Source: CAD feature listing. Evaluate the final solid. Frame: model axes, mm. Give positions to 0.01 mm unless a question says otherwise; leave off trailing zeros. Order: outer loops, then holes, each group sorted by start corner. A loop starts at its lowest first (then second) coordinate and runs counter-clockwise, first axis right, second up. Notation, with made-up numbers: M -7,66.5 L 2,66.5 A20 cw 2,93.5 Z; hole C 57,71.25 d6. An arc over 180 degrees is marked long. Answer as a JSON object with one key per item and string values. Group by question number.
1. Section query C-C (x = -66.5). Output: boundary loops of the cut face in (y, z), plus the area to 3 significant figures.
2. Material intervals for L1, parallel to Y at x = 31.5, z = 1.75; L2, parallel to Y at x = 16, z = 1.35; L3, parallel to Y at x = 50, z = 0.55, sorted ascending. Write a range as [from, to].
3. Pin query (flat end, axial travel): P1, Ø1.5, axis at y = 150, z = 1.5, coming from the -X side; P2, Ø1.7, axis at y = 218, z = 1, coming from the -X side. Return the tip coordinate at first contact, or that it passes through.
4. Section query A-A (y = 34.03). Output: boundary loops of the cut face in (x, z) (3 decimals).
5. Section query B-B (z = 1.5). Count the separate pieces of the cut face and the enclosed holes in it, plus the area to 3 significant figures.
from build123d import *

# Parameters (mm, degrees)
MODEL_R             = 3.6
MODEL_R_2           = 2.5
BOSS_EXTRUDE1_DEPTH = 3


with BuildPart() as part:
    # Model → Boss-Extrude1 (new body)
    with BuildSketch(Plane.XY):
        with BuildLine():
            Line((-86.64, 0), (86.64, 0))
            ThreePointArc((86.64, 0), (89.015878785, 0.984121215), (90, 3.36))
            Line((90, 3.36), (90, 217.83))
            ThreePointArc((90, 217.83), (87.167722574, 224.667722574), (80.33, 227.5))
            Line((80.33, 227.5), (-19.67, 227.5))
            ThreePointArc((-19.67, 227.5), (-25.584006957, 225.942971908), (-29.964579281, 221.67560728))
            Line((-29.964579281, 221.67560728), (-86.618767522, 127.387204203))
            ThreePointArc((-86.618767522, 127.387204203), (-89.126906327, 120.031940724), (-90, 112.31))
            Line((-90, 112.31), (-90, 3.36))
            ThreePointArc((-90, 3.36), (-89.015878785, 0.984121215), (-86.64, 0))
        make_face()
        with Locations((-75.285, 13.33)):
            Circle(MODEL_R, mode=Mode.SUBTRACT)
        with Locations((-7.295, 209.94)):
            Circle(MODEL_R_2, mode=Mode.SUBTRACT)
        with Locations((-7.295, 189.94)):
            Circle(MODEL_R_2, mode=Mode.SUBTRACT)
        with Locations((-7.295, 169.94)):
            Circle(MODEL_R_2, mode=Mode.SUBTRACT)
        with Locations((-35.285, 113.03)):
            Circle(MODEL_R_2, mode=Mode.SUBTRACT)
        with Locations((-75.285, 113.03)):
            Circle(MODEL_R_2, mode=Mode.SUBTRACT)
        with Locations((75.315, 13.33)):
            Circle(MODEL_R, mode=Mode.SUBTRACT)
        with Locations((0, 13.33)):
            Circle(MODEL_R, mode=Mode.SUBTRACT)
        with Locations((56.355, 34.03)):
            Circle(MODEL_R_2, mode=Mode.SUBTRACT)
        with Locations((53.705, 189.94)):
            Circle(MODEL_R_2, mode=Mode.SUBTRACT)
        with Locations((73.365, 165.98)):
            Circle(MODEL_R_2, mode=Mode.SUBTRACT)
        with Locations((73.365, 145.98)):
            Circle(MODEL_R_2, mode=Mode.SUBTRACT)
        with Locations((52.865, 145.98)):
            Circle(MODEL_R_2, mode=Mode.SUBTRACT)
        with Locations((56.355, 129.03)):
            Circle(MODEL_R_2, mode=Mode.SUBTRACT)
        with Locations((75.315, 113.03)):
            Circle(MODEL_R_2, mode=Mode.SUBTRACT)
        with Locations((35.315, 113.03)):
            Circle(MODEL_R_2, mode=Mode.SUBTRACT)
        with BuildLine():
            Line((-26.095, 100.21), (-26.095, 109.21))
            ThreePointArc((-26.095, 109.21), (-23.555, 111.75), (-21.015, 109.21))
            Line((-21.015, 109.21), (-21.015, 100.21))
            ThreePointArc((-21.015, 100.21), (-23.555, 97.67), (-26.095, 100.21))
        make_face(mode=Mode.SUBTRACT)
        with BuildLine():
            Line((-26.095, 147.35), (-26.095, 156.35))
            ThreePointArc((-26.095, 156.35), (-23.555, 158.89), (-21.015, 156.35))
            Line((-21.015, 156.35), (-21.015, 147.35))
            ThreePointArc((-21.015, 147.35), (-23.555, 144.81), (-26.095, 147.35))
        make_face(mode=Mode.SUBTRACT)
        with BuildLine():
            Line((21.045, 100.21), (21.045, 109.21))
            ThreePointArc((21.045, 109.21), (23.585, 111.75), (26.125, 109.21))
            Line((26.125, 109.21), (26.125, 100.21))
            ThreePointArc((26.125, 100.21), (23.585, 97.67), (21.045, 100.21))
        make_face(mode=Mode.SUBTRACT)
        with BuildLine():
            Line((21.045, 147.35), (21.045, 156.35))
            ThreePointArc((21.045, 156.35), (23.585, 158.89), (26.125, 156.35))
            Line((26.125, 156.35), (26.125, 147.35))
            ThreePointArc((26.125, 147.35), (23.585, 144.81), (21.045, 147.35))
        make_face(mode=Mode.SUBTRACT)
        with BuildLine():
            Line((27.205, 216.97), (27.205, 219.09))
            ThreePointArc((27.205, 219.09), (27.626766235, 220.108233765), (28.645, 220.53))
            Line((28.645, 220.53), (37.765, 220.53))
            ThreePointArc((37.765, 220.53), (38.783233765, 220.108233765), (39.205, 219.09))
            Line((39.205, 219.09), (39.205, 216.97))
            ThreePointArc((39.205, 216.97), (38.783233765, 215.951766235), (37.765, 215.53))
            Line((37.765, 215.53), (28.645, 215.53))
            ThreePointArc((28.645, 215.53), (27.626766235, 215.951766235), (27.205, 216.97))
        make_face(mode=Mode.SUBTRACT)
        with BuildLine():
            Line((76.385, 175.96), (75.817986625, 175.249714613))
            add(Edge.make_bspline(
                [(70.912013375, 175.249714613), (70.912013375, 172.796727988), (73.365, 172.796727988), (75.817986625, 172.796727988), (75.817986625, 175.249714613)],
                knots=[3.141592654, 3.141592654, 3.141592654, 4.71238898, 4.71238898, 6.283185307, 6.283185307, 6.283185307], degree=2, weights=[1, 0.707106781, 1, 0.707106781, 1]))
            Line((70.912013375, 175.249714613), (69.945, 176.461071346))
            Line((69.945, 176.461071346), (67.475, 176.461071346))
            ThreePointArc((67.475, 176.461071346), (66.301202743, 176.947274089), (65.815, 178.121071346))
            Line((65.815, 178.121071346), (65.815, 190.45))
            ThreePointArc((65.815, 190.45), (66.301202743, 191.623797257), (67.475, 192.11))
            Line((67.475, 192.11), (78.855, 192.11))
            ThreePointArc((78.855, 192.11), (80.028797257, 191.623797257), (80.515, 190.45))
            Line((80.515, 190.45), (80.515, 177.62))
            ThreePointArc((80.515, 177.62), (80.028797257, 176.446202743), (78.855, 175.96))
            Line((78.855, 175.96), (76.385, 175.96))
        make_face(mode=Mode.SUBTRACT)
        with BuildLine():
            Line((47.015, 205.17), (47.015, 214.86))
            ThreePointArc((47.015, 214.86), (47.934684707, 217.080315293), (50.155, 218))
            Line((50.155, 218), (74.165, 218))
            ThreePointArc((74.165, 218), (78.655128061, 216.140128061), (80.515, 211.65))
            Line((80.515, 211.65), (80.515, 205.17))
            ThreePointArc((80.515, 205.17), (79.595315293, 202.949684707), (77.375, 202.03))
            Line((77.375, 202.03), (50.155, 202.03))
            ThreePointArc((50.155, 202.03), (47.934684707, 202.949684707), (47.015, 205.17))
        make_face(mode=Mode.SUBTRACT)
        with BuildLine():
            Line((33.205, 167.44), (12.205, 167.44))
            ThreePointArc((12.205, 167.44), (9.705, 169.94), (12.205, 172.44))
            Line((12.205, 172.44), (33.205, 172.44))
            ThreePointArc((33.205, 172.44), (35.705, 169.94), (33.205, 167.44))
        make_face(mode=Mode.SUBTRACT)
        with BuildLine():
            Line((33.205, 187.44), (12.205, 187.44))
            ThreePointArc((12.205, 187.44), (9.705, 189.94), (12.205, 192.44))
            Line((12.205, 192.44), (33.205, 192.44))
            ThreePointArc((33.205, 192.44), (35.705, 189.94), (33.205, 187.44))
        make_face(mode=Mode.SUBTRACT)
        with BuildLine():
            Line((33.205, 207.44), (12.205, 207.44))
            ThreePointArc((12.205, 207.44), (9.705, 209.94), (12.205, 212.44))
            Line((12.205, 212.44), (33.205, 212.44))
            ThreePointArc((33.205, 212.44), (35.705, 209.94), (33.205, 207.44))
        make_face(mode=Mode.SUBTRACT)
        with BuildLine():
            Line((-12.5, 123.28), (-12.5, 133.28))
            ThreePointArc((-12.5, 133.28), (0, 145.78), (12.5, 133.28))
            Line((12.5, 133.28), (12.5, 123.28))
            ThreePointArc((12.5, 123.28), (0, 110.78), (-12.5, 123.28))
        make_face(mode=Mode.SUBTRACT)
    extrude(amount=BOSS_EXTRUDE1_DEPTH)


solid = part.part
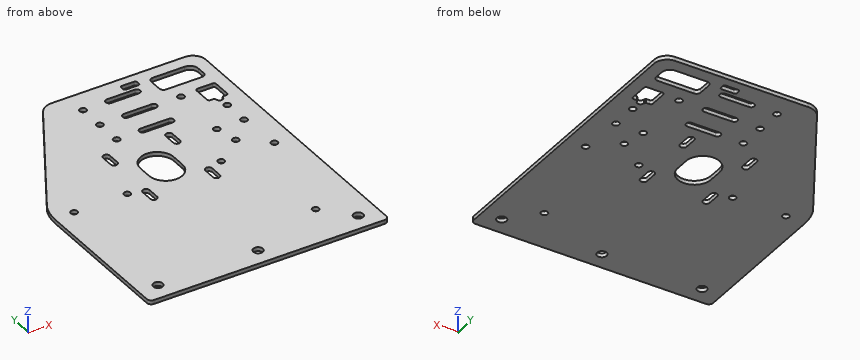
Answer sheet:
{
 "1": {"outline": "M 0,0 L 160.87,0 L 160.87,3 L 0,3 Z", "area": "483 mm^2"},
 "2": {"L1": "[0, 167.44], [172.44, 187.44], [192.44, 207.44], [212.44, 215.53], [220.53, 227.5]", "L2": "[0, 167.44], [172.44, 187.44], [192.44, 207.44], [212.44, 227.5]", "L3": "[0, 202.03], [218, 227.5]"},
 "3": {"P1": "x = -73.48", "P2": "x = -32.68"},
 "4": {"outline": "M -90,0 L 53.855,0 L 53.855,3 L -90,3 Z; M 58.855,0 L 90,0 L 90,3 L 58.855,3 Z"},
 "5": {"separate pieces": "1", "enclosed holes": "27", "area": "35,000 mm^2"}
}
